Geometry check sheet. Reference: the model listing, model coordinates, mm. Face numbers are marked on the shaded views. A direction names the side the tool comes from. Give positions to 0.01 mm unless a question says otherwise; leave off trailing zeros. Order: outer loops, then holes, each group sorted by start corner. A loop starts at its lowest first (then second) coordinate and runs counter-clockwise, first axis right, second up.
from build123d import *

# Parameters (mm, degrees)
SKETCH1_R           = 4.75
BOSS_EXTRUDE1_DEPTH = 13
SKETCH2_R           = 12
BOSS_EXTRUDE2_DEPTH = 2
CHAMFER1_SIZE       = 2
CUT_EXTRUDE1_START  = -12
CUT_EXTRUDE1_DEPTH  = 12
BOSS_EXTRUDE3_DEPTH = 2
CHAMFER3_SIZE       = 6
CHAMFER3_SIZE_2     = 1.057961884
CHAMFER4_SIZE       = 1


# Some blends are built 0.0001 mm under size
with BuildPart() as part:
    # Sketch1 → Boss-Extrude1 (new body)
    with BuildSketch(Plane(origin=(0, 0, 0), x_dir=(1, 0, 0), z_dir=(0, 1, 0))):
        with Locations(Location((0, 0, 0), (0, 0, 90))):
            Circle(SKETCH1_R)
    extrude(amount=BOSS_EXTRUDE1_DEPTH)

    # Sketch2 → Boss-Extrude2 (add)
    with BuildSketch(Plane.XZ):
        with Locations(Location((0, 0, 0), (0, 0, 270))):
            Circle(SKETCH2_R)
    extrude(amount=BOSS_EXTRUDE2_DEPTH)

    # Chamfer1
    chamfer1_edges = [part.edges().sort_by_distance(p)[0] for p in [
        (0, -2, 12),
    ]]
    chamfer(chamfer1_edges, length=CHAMFER1_SIZE - 0.0001)  # a hair under: the kernel refuses the full size

    # Sketch4 → Cut-Extrude1 (cut)
    with BuildSketch(Plane(origin=(0, 13, 0), x_dir=(1, 0, 0), z_dir=(0, 1, 0)).offset(CUT_EXTRUDE1_START)):
        with BuildLine():
            Line((-0.989583333, -4.645774944), (-0.989583333, 4.645774944))
            ThreePointArc((-0.989583333, 4.645774944), (0, 4.75), (0.989583333, 4.645774944))
            Line((0.989583333, 4.645774944), (0.989583333, -4.645774944))
            ThreePointArc((0.989583333, -4.645774944), (0, -4.75), (-0.989583333, -4.645774944))
        make_face()
    extrude(amount=CUT_EXTRUDE1_DEPTH, mode=Mode.SUBTRACT)

    # Sketch5 → Boss-Extrude3 (add)
    with BuildSketch(Plane(origin=(0, 13, 0), x_dir=(1, 0, 0), z_dir=(0, 1, 0))):
        with BuildLine():
            Line((1.197916667, -4.645774944), (3.388107905, -4.645774944))
            ThreePointArc((3.388107905, -4.645774944), (5.75, 0), (3.388107905, 4.645774944))
            Line((3.388107905, 4.645774944), (1.197916667, 4.645774944))
            Line((1.197916667, 4.645774944), (0.989583333, 4.645774944))
            Line((0.989583333, 4.645774944), (0.989583333, -4.645774944))
            Line((0.989583333, -4.645774944), (1.197916667, -4.645774944))
        make_face()
        with BuildLine():
            Line((-1.197916667, -4.645774944), (-3.388107905, -4.645774944))
            ThreePointArc((-3.388107905, -4.645774944), (-5.75, 0), (-3.388107905, 4.645774944))
            Line((-3.388107905, 4.645774944), (-1.197916667, 4.645774944))
            Line((-1.197916667, 4.645774944), (-0.989583333, 4.645774944))
            Line((-0.989583333, 4.645774944), (-0.989583333, -4.645774944))
            Line((-0.989583333, -4.645774944), (-1.197916667, -4.645774944))
        make_face()
    extrude(amount=-BOSS_EXTRUDE3_DEPTH)

    # Chamfer3
    # the kernel refuses this chamfer: 6, 1.057961884 mm, written as the material it adds along each edge
    with BuildSketch(Plane(origin=(0, 11, 0), x_dir=(-0.9999950652018581, 0, -0.0031415874858794902), z_dir=(-0.0031415874858794902, 0, 0.9999950652018581))) as chamfer3_piece_1_section:
        Polygon((4.75, CHAMFER3_SIZE), (4.75 + CHAMFER3_SIZE_2, 0), (4.75, 0), align=None)
    chamfer3_piece_1 = revolve(axis=Axis((0, 11, 0), (0, -1, 0)), revolution_arc=359.64, mode=Mode.PRIVATE)
    chamfer3_piece_1 = split(chamfer3_piece_1, bisect_by=Plane(origin=(-4.007024844, 8.962519636, 4.645774944), z_dir=(0, 0, -1)), keep=Keep.TOP, mode=Mode.PRIVATE)
    chamfer3_piece_1 = split(chamfer3_piece_1, bisect_by=Plane(origin=(-4.007024844, 8.962519636, -4.645774944), z_dir=(0, 0, 1)), keep=Keep.TOP, mode=Mode.PRIVATE)
    chamfer3_piece_1 = chamfer3_piece_1 & Plane(origin=(0, 8.962519636, 0), x_dir=(0.5892361573319569, 0, 0.8079608597529149), z_dir=(0, 1, 0)) * Cylinder(5.75, 24, mode=Mode.PRIVATE)
    add(chamfer3_piece_1)
    with BuildSketch(Plane(origin=(0, 11, 0), x_dir=(0.9999950652018581, 0, 0.003141587485879146), z_dir=(0.003141587485879146, 0, -0.9999950652018581))) as chamfer3_piece_2_section:
        Polygon((4.75, CHAMFER3_SIZE), (4.75 + CHAMFER3_SIZE_2, 0), (4.75, 0), align=None)
    chamfer3_piece_2 = revolve(axis=Axis((0, 11, 0), (0, -1, 0)), revolution_arc=359.64, mode=Mode.PRIVATE)
    chamfer3_piece_2 = split(chamfer3_piece_2, bisect_by=Plane(origin=(4.007024844, 8.962519636, 4.645774944), z_dir=(0, 0, -1)), keep=Keep.TOP, mode=Mode.PRIVATE)
    chamfer3_piece_2 = split(chamfer3_piece_2, bisect_by=Plane(origin=(4.007024844, 8.962519636, -4.645774944), z_dir=(0, 0, 1)), keep=Keep.TOP, mode=Mode.PRIVATE)
    chamfer3_piece_2 = chamfer3_piece_2 & Plane(origin=(0, 8.962519636, 0), x_dir=(0.5892361573319569, 0, 0.8079608597529149), z_dir=(0, 1, 0)) * Cylinder(5.75, 24, mode=Mode.PRIVATE)
    add(chamfer3_piece_2)

    # Chamfer4
    chamfer4_edges = [part.edges().sort_by_distance(p)[0] for p in [
        (5.75, 13, 0),
        (-5.75, 13, 0),
    ]]
    chamfer(chamfer4_edges, length=CHAMFER4_SIZE)


solid = part.part
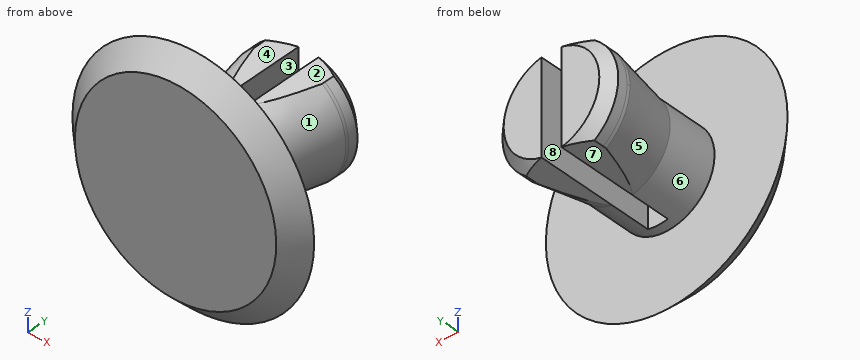
Item 1: Sectioned sample at B-B (y = 5.5). Enter the section's corners in (x, z), and give its area (3 significant figures).
Reported:
outline: (-1.35, -4.65) - (-0.99, -4.65) - (-0.99, 4.65) - (-1.35, 4.65) arc R4.84 ccw to start; (0.99, -4.65) - (1.35, -4.65) arc R4.84 ccw to (1.35, 4.65) - (0.99, 4.65) - close
area: 54.5 mm2
Item 2: Draft check along X on the marked faces 1, 2 and 3. Enter one of: released by +X, released by -X, zero draft, split by the parting line, or undercut.
Reported:
face 1: released by +X
face 2: zero draft
face 3: undercut
Item 3: Scan lines: L1, parallel to X at y = 2, z = -1; L2, parallel to Y at x = 0, z = -8.5; L3, parallel to X at y = 4, z = -2.5. Record each from-to range of solid material in increasing order.
Reported:
L1: x = -4.64 to -0.99, 0.99 to 4.64
L2: y = -2 to 0
L3: x = -4.04 to -0.99, 0.99 to 4.04
Item 4: Gauge pin test, flat ends, axial feed: pin 1 (1 mm diameter, centred on y = 11.5, z = -2.5, fed in from +X); pin 2 (2.5 mm diameter, centred on x = 3, y = 8.5, fed in from -Z); pin 3 (2.5 mm diameter, centred on x = 2, y = 7.5, fed in from +Z); pin 4 (7 mm diameter, centred on x = 0, z = -5, fed in from +Y). Record the tip position at first contact, or that the pin passes through.
Reported:
pin 1: stops at x = 5.39
pin 2: stops at z = -4.65
pin 3: stops at z = 4.65
pin 4: stops at y = 13
Item 5: Set-up check for the marked faces 4, 5, 6, 7 and 8: record each of +Z, -Z, +X, -X, +Y, -Y from which the full face is reachable in a straight line by a thin tool's end or side.
Reported:
face 4: +Z, +X, -X, +Y
face 5: -X
face 6: none
face 7: -Z, +X, -X, +Y
face 8: +Z, -Z, +Y
